Autodesk Inventor part; units mm, degrees
ref_plane "YZ Plane" through (0, 0, 0) normal (1, 0, 0) x (0, 1, 0)
ref_plane "XZ Plane" through (0, 0, 0) normal (0, 1, 0) x (-1, 0, 0)
ref_plane "XY Plane" through (0, 0, 0) normal (0, 0, 1) x (1, 0, 0)
sketch "Sketch1" plane through (0, 0, 0) normal (0, 0, 1) x (1, 0, 0)
  circle A0 centre (0, 0) radius 160
  circle A1 centre (0, 0) radius 150
  line L0 (0, 0) -> (0, -160) construction
  dimension "outer_diameter" = 320
  dimension "inner_diameter" = 300
extrude "Extrusion1" add sketch "Sketch1" along normal blind 5
sketch "Sketch2" plane through (0, 0, 5) normal (0, 0, 1) x (1, 0, 0)
  arc A0 (136.8569, 72.7681) -> (0, 155) centre (0, 0) ccw construction
  arc A1 (139.285, 74.0591) -> (0, 157.75) centre (0, 0) ccw
  arc A2 (134.4288, 71.477) -> (0, 152.25) centre (0, 0) ccw
  arc A3 (134.4288, 71.477) -> (139.285, 74.0591) centre (136.8569, 72.7681) ccw
  arc A4 (0, 157.75) -> (0, 152.25) centre (0, 155) ccw
  line L0 (0, 0) -> (136.8569, 72.7681) construction
  line L1 (0, 0) -> (0, 155) construction
  line L2 (0, 0) -> (0, -28.237) construction
  arc A5 (-27.393, 155.3534) -> (-150.0292, 48.7474) centre (0, 0) ccw
  arc A6 (-26.4379, 149.937) -> (-144.7984, 47.0478) centre (0, 0) ccw
  arc A7 (-26.4379, 149.937) -> (-27.393, 155.3534) centre (-26.9155, 152.6452) ccw
  arc A8 (-150.0292, 48.7474) -> (-144.7984, 47.0478) centre (-147.4138, 47.8976) ccw
  arc A9 (-156.2148, 21.9546) -> (-92.7231, -127.6224) centre (0, 0) ccw
  arc A10 (-150.7683, 21.1891) -> (-89.4903, -123.1728) centre (0, 0) ccw
  arc A11 (-150.7683, 21.1891) -> (-156.2148, 21.9546) centre (-153.4916, 21.5718) ccw
  arc A12 (-92.7231, -127.6224) -> (-89.4903, -123.1728) centre (-91.1067, -125.3976) ccw
  arc A13 (-69.153, -141.7848) -> (92.7231, -127.6224) centre (0, 0) ccw
  arc A14 (-66.742, -136.8414) -> (89.4903, -123.1728) centre (0, 0) ccw
  arc A15 (-66.742, -136.8414) -> (-69.153, -141.7848) centre (-67.9475, -139.3131) ccw
  arc A16 (92.7231, -127.6224) -> (89.4903, -123.1728) centre (91.1067, -125.3976) ccw
  arc A17 (113.4759, -109.5824) -> (150.0292, 48.7474) centre (0, 0) ccw
  arc A18 (109.5195, -105.7617) -> (144.7984, 47.0478) centre (0, 0) ccw
  arc A19 (109.5195, -105.7617) -> (113.4759, -109.5824) centre (111.4977, -107.672) ccw
  arc A20 (150.0292, 48.7474) -> (144.7984, 47.0478) centre (147.4138, 47.8976) ccw
  point P0 (160, 0)
  dimension "slot_radius" = 155
  dimension "slot_length_deg" = 62
  dimension "slot_width" = 5.5
  dimension "d15" = 360
extrude "Extrusion3" cut sketch "Sketch2" against normal blind 5
sketch "Sketch3" plane through (0, 0, 5) normal (0, 0, 1) x (1, 0, 0)
  circle A0 centre (0, 0) radius 150
  circle A1 centre (0, 0) radius 155 construction
  line L0 (0, 0) -> (-13.5091, 154.4102) construction
  arc A2 (0, 157.75) -> (0, 152.25) centre (0, 155) ccw
  line L1 (0, 155) -> (0, 0) construction
  point P0 (-13.5091, 154.4102)
  point P1 (-151.0274, 34.8674)
  point P2 (-79.8309, -132.8609)
  point P3 (101.6891, -116.98)
  point P4 (142.6783, 60.5633)
  dimension "d22" = 310
  dimension "d42" = 360
  dimension "d52" = 5
hole "Hole1" at (-13.5091, 154.4102, 5) at (-151.0274, 34.8674, 5) at (-79.8309, -132.8609, 5) at (101.6891, -116.98, 5) at (142.6783, 60.5633, 5) direction (0, 0, -1) diameter 4.134 depth 8 tip angle 118
equation "\"slot_radius\" = 0.25 * inner_diameter + 0.25 * outer_diameter"
equation "\"d17\" = thickness"
equation "\"d22\" = 0.5 * inner_diameter + 0.5 * outer_diameter"
equation "\"offset_angle_gear\" = 65deg"
properties part number "ytterring"
Work out the finished part from the listing and answer in its coordinate system (mm). A direction names the side the tool comes from. Coordinates: 2 decimals unless noted, no trailing zeros. Loops run counter-clockwise (first coordinate to the right, second up) from the corner with the lowest first, then second, coordinate; pieces in that order, holes last. Notation, with made-up numbers: M 61.5,-4 L 79.5,-4 A34 ccw 79.5,34 Z; hole C 34.5,86 d6. An arc over 180 degrees is marked long. Answer in a Markdown table with one row per item. Add a question column.
1. A flat-ended cylindrical pin translates along its axis: P1, Ø3.5, axis at x = 142.68, y = 60.56, coming from the +Z side. Find the tip coordinate at first contact, or state that the pin passes through.
2. Find section C-C, the plane y = 79. Write down the section's boundary in (x, z), then the cut area to 3 significant figures.
3. Consider L1, parallel to X at y = -121, z = 2.05; L2, parallel to Y at x = 59.5, z = 2.35; L3, parallel to Y at x = -68, z = 3.15. Determine where each line is inside the solid, lowest interval first.
4. The mould has two halves that part along X. Classify faces 1 (the flat face through (-143, 48, 5)), 2 (the cylindrical face through (12.56, -157.25, 2.54)), 3 (the cylindrical face through (-34.685, 156.195, 2.465)), 4 (the cylindrical face through (-19.527, -148.724, 2.465)): pulls with the +X half, pulls with the -X half, needs draft (parallel to the pull), parting line crosses it, or undercut.
5. Find section B-B, the plane z = 0.9. State how many separate pieces and enclosed holes the cut face has, then the cut area to 3 significant figures.
6. Find section A-A, the plane y = 0. Write down the section's boundary in (x, z).
7. A tool of negligible diameter and unlimited length cuts with its end or side. For faces 5 (the cylindrical face through (82.27, 134.6, 2.54)), 6 (the flat face through (-143, 48, 0)), from which of +Z, -Z, +X, -X, +Y, -Y can it reach the whole face along a straight path? Write none if from no direction.
Reported:
| question | item | result |
|---|---|---|
| 1 | P1 | passes through |
| 2 | outline | M -139.14,0 L -136.54,0 L -136.54,5 L -139.14,5 Z; M -130.15,0 L -127.51,0 L -127.51,5 L -130.15,5 Z; M 127.51,0 L 130.15,0 L 130.15,5 L 127.51,5 Z; M 136.54,0 L 139.14,0 L 139.14,5 L 136.54,5 Z |
| 2 | area | 52.3 mm^2 |
| 3 | L1 | x = -104.69 to -101.21, -92.41 to -88.65, 88.65 to 104.69 |
| 3 | L2 | y = -148.53 to -146.1, -140.14 to -137.69, 137.69 to 140.14, 146.1 to 148.53 |
| 3 | L3 | y = -144.83 to -142.34, -136.56 to -133.7, 133.7 to 136.22, 142.34 to 144.83 |
| 4 | face 1 | needs draft |
| 4 | face 2 | undercut |
| 4 | face 3 | parting line crosses it |
| 4 | face 4 | undercut |
| 5 | separate pieces | 1 |
| 5 | enclosed holes | 11 |
| 5 | area | 4,940 mm^2 |
| 6 | outline | M -160,0 L -157.75,0 L -157.75,5 L -160,5 Z; M -152.25,0 L -150,0 L -150,5 L -152.25,5 Z; M 150,0 L 152.25,0 L 152.25,5 L 150,5 Z; M 157.75,0 L 160,0 L 160,5 L 157.75,5 Z |
| 7 | face 5 | +Z, -Z |
| 7 | face 6 | -Z, +X, -X, +Y, -Y |
